Geometry check sheet. Reference: the model listing, model coordinates, mm. Round coordinates to 2 decimals unless told otherwise and drop trailing zeros. Order: outer loops, then holes, each group sorted by start corner. A loop starts at its lowest first (then second) coordinate and runs counter-clockwise, first axis right, second up. Notation, with made-up numbers: (66, -16.5) - (71, -16.5) arc R32 cw to (71, 16.5) - close; hole circle Ø4 at (38.5, 21.5). An arc over 180 degrees is marked (long way). Return JSON: item names as keys, results as strings. Group by question number.
Q1. Sectioned sample at B-B, the plane z = 30. Give the number of separate pieces and of enclosed holes in the cut face, then the cut area to 3 significant figures.
Q2. Draft check along X on faces 1 (the cylindrical face through (83.672, -14.965, 25.35)), 2 (the flat face through (-1, 2, 0)). Enter one of: pulls with the +X half, pulls with the -X half, needs draft (parallel to the pull), parting line crosses it, or undercut.
Q3. Gauge pin test, flat ends, axial feed: pin 1 Ø3 at (x, z) = (-26.5, 14) entering from -Y; pin 2 Ø3 at (x, y) = (-79, 12.5) entering from +Z; pin 3 Ø12 at (x, z) = (48.5, 23.5) entering from +Y. Record the tip position at first contact, or that the pin passes through.
Q4. Sectioned sample at A-A, the plane x = 0. Record the cut outline in (y, z).
Q5. Material ranges on line 1 along Y through (x, z) = (40, 40.5); line 2 along Y through (x, z) = (68.5, 45); line 3 along Y through (x, z) = (19, 28.5), recorded low to high.
```python
from build123d import *

# Parameters (mm, degrees)
SKETCH_1_R          = 100
EXTRUDE_1_DEPTH     = 50
SKETCH_2_R          = 10
EXTRUDE_2_DEPTH     = 50
FILLET_1_R          = 15
CUT_EXTRUDE_1_DEPTH = 151.000000067


with BuildPart() as part:
    # 草图1 → 凸台-拉伸1 (new body)
    with BuildSketch(Plane.XY):
        Circle(SKETCH_1_R)
    extrude(amount=EXTRUDE_1_DEPTH)

    # 草图2 → 凸台-拉伸2 (add)
    with BuildSketch(Plane.XY.offset(50)):
        Circle(SKETCH_2_R)
    extrude(amount=EXTRUDE_2_DEPTH)

    # 圆角1
    fillet_1_edges = [part.edges().sort_by_distance(p)[0] for p in [
        (-100, 0, 0),
        (-100, 0, 50),
    ]]
    fillet(fillet_1_edges, radius=FILLET_1_R)

    # 草图3 → 切除-拉伸1 (cut, through all)
    with BuildSketch(Plane.XY.offset(50)):
        with BuildLine():
            ThreePointArc((-11.262655322, 19.507491245), (-7.704109975, 21.166868192), (-3.911479145, 22.18310056))
            Line((-3.911479145, 22.18310056), (-14.760095102, 83.708659006))
            ThreePointArc((-14.760095102, 83.708659006), (-29.071712183, 79.873872767), (-42.5, 73.612159322))
            Line((-42.5, 73.612159322), (-11.262655322, 19.507491245))
        make_face()
        with BuildLine():
            Line((14.760095102, 83.708659006), (3.911479145, 22.18310056))
            ThreePointArc((3.911479145, 22.18310056), (7.704109975, 21.166868192), (11.262655322, 19.507491245))
            Line((11.262655322, 19.507491245), (42.5, 73.612159322))
            ThreePointArc((42.5, 73.612159322), (29.071712183, 79.873872767), (14.760095102, 83.708659006))
        make_face()
        with BuildLine():
            Line((65.113777665, 54.636946823), (17.255389048, 14.478990586))
            ThreePointArc((17.255389048, 14.478990586), (19.507491245, 11.262655322), (21.166868192, 7.704109975))
            Line((21.166868192, 7.704109975), (79.873872767, 29.071712183))
            ThreePointArc((79.873872767, 29.071712183), (73.612159322, 42.5), (65.113777665, 54.636946823))
        make_face()
        with BuildLine():
            Line((85, 0), (22.525310643, 0))
            ThreePointArc((22.525310643, 0), (22.18310056, -3.911479145), (21.166868192, -7.704109975))
            Line((21.166868192, -7.704109975), (79.873872767, -29.071712183))
            ThreePointArc((79.873872767, -29.071712183), (83.708659006, -14.760095102), (85, 0))
        make_face()
        with BuildLine():
            Line((65.113777665, -54.636946823), (17.255389048, -14.478990586))
            ThreePointArc((17.255389048, -14.478990586), (14.478990586, -17.255389048), (11.262655322, -19.507491245))
            Line((11.262655322, -19.507491245), (42.5, -73.612159322))
            ThreePointArc((42.5, -73.612159322), (54.636946823, -65.113777665), (65.113777665, -54.636946823))
        make_face()
        with BuildLine():
            Line((14.760095102, -83.708659006), (3.911479145, -22.18310056))
            ThreePointArc((3.911479145, -22.18310056), (0, -22.525310643), (-3.911479145, -22.18310056))
            Line((-3.911479145, -22.18310056), (-14.760095102, -83.708659006))
            ThreePointArc((-14.760095102, -83.708659006), (0, -85), (14.760095102, -83.708659006))
        make_face()
        with BuildLine():
            Line((-42.5, -73.612159322), (-11.262655322, -19.507491245))
            ThreePointArc((-11.262655322, -19.507491245), (-14.478990586, -17.255389048), (-17.255389048, -14.478990586))
            Line((-17.255389048, -14.478990586), (-65.113777665, -54.636946823))
            ThreePointArc((-65.113777665, -54.636946823), (-54.636946823, -65.113777665), (-42.5, -73.612159322))
        make_face()
        with BuildLine():
            Line((-79.873872767, -29.071712183), (-21.166868192, -7.704109975))
            ThreePointArc((-21.166868192, -7.704109975), (-22.18310056, -3.911479145), (-22.525310643, 0))
            Line((-22.525310643, 0), (-85, 0))
            ThreePointArc((-85, 0), (-83.708659006, -14.760095102), (-79.873872767, -29.071712183))
        make_face()
        with BuildLine():
            Line((-79.873872767, 29.071712183), (-21.166868192, 7.704109975))
            ThreePointArc((-21.166868192, 7.704109975), (-19.507491245, 11.262655322), (-17.255389048, 14.478990586))
            Line((-17.255389048, 14.478990586), (-65.113777665, 54.636946823))
            ThreePointArc((-65.113777665, 54.636946823), (-73.612159322, 42.5), (-79.873872767, 29.071712183))
        make_face()
    extrude(amount=-CUT_EXTRUDE_1_DEPTH, mode=Mode.SUBTRACT)


solid = part.part
```
Reply:
{
 "1": {"separate pieces": "1", "enclosed holes": "9", "area": "20,900 mm^2"},
 "2": {"face 1": "undercut", "face 2": "needs draft"},
 "3": {"pin 1": "y = -96.8", "pin 2": "z = 50", "pin 3": "y = 90.52"},
 "4": {"outline": "(-100, 15) arc R15 ccw to (-85, 0) - (-85, 50) arc R15 ccw to (-100, 35) - close; (-22.53, 0) - (85, 0) arc R15 ccw to (100, 15) - (100, 35) arc R15 ccw to (85, 50) - (10, 50) - (10, 100) - (-10, 100) - (-10, 50) - (-22.53, 50) - close"},
 "5": {"line 1": "-90.51 to -69.28, -33.56 to -14.56, 0 to 14.56, 33.56 to 69.28, 75 to 90.51", "line 2": "-67.52 to -24.93, 0 to 24.93, 50.33 to 67.52", "line 3": "-98.18 to -32.91, -15.94 to 12.1, 15.94 to 32.91, 82.85 to 98.18"}
}
